```python
from build123d import *

# Parameters (mm, degrees)
BOSS_EXTRUDE1_DEPTH      = 1
F_4_0_4_DIAMETER_HOLE3_D = 4
F_4_0_4_DIAMETER_HOLE2_D = 4
CUT_EXTRUDE1_DEPTH       = 185.301435156
F_4_0_4_DIAMETER_HOLE1_D = 4
LPATTERN1_COUNT          = 10
LPATTERN1_PITCH          = 10
FILLET1_R                = 4


with BuildPart() as part:
    # Sketch1 → Boss-Extrude1 (new body)
    with BuildSketch(Plane(origin=(0, 0, 0), x_dir=(0, 0, -1), z_dir=(1, 0, 0))):
        with BuildLine():
            Line((12, -183), (12, -85))
            ThreePointArc((12, -85), (21.475099597, -58.206374501), (18, -30))
            Line((18, -30), (18, 0))
            Line((18, 0), (-18, 0))
            Line((-18, 0), (-18, -30))
            ThreePointArc((-18, -30), (-21.475099597, -58.206374501), (-12, -85))
            Line((-12, -85), (-12, -183))
            Line((-12, -183), (12, -183))
        make_face()
    extrude(amount=BOSS_EXTRUDE1_DEPTH)

    # Ø4.0 (4) Diameter Hole3 (through all)
    with Locations(Plane.ZY):
        with Locations((10, -10), (-10, -10)):
            Hole(F_4_0_4_DIAMETER_HOLE3_D / 2)

    # Ø4.0 (4) Diameter Hole2 (through all)
    with Locations(Plane.ZY):
        with Locations((-13, -19), (13, -19)):
            Hole(F_4_0_4_DIAMETER_HOLE2_D / 2)

    # Sketch10 → Cut-Extrude1 (cut, through all)
    with BuildSketch(Plane(origin=(1, 0, 0), x_dir=(0, 0, -1), z_dir=(1, 0, 0))):
        with BuildLine():
            Line((-2, -15), (2, -15))
            ThreePointArc((2, -15), (3, -16), (2, -17))
            Line((2, -17), (-2, -17))
            ThreePointArc((-2, -17), (-3, -16), (-2, -15))
        make_face()
    extrude(amount=-CUT_EXTRUDE1_DEPTH, mode=Mode.SUBTRACT)

    # Ø4.0 (4) Diameter Hole1 (through all)
    with Locations(Plane(origin=(1, 0, 0), x_dir=(0, 0, -1), z_dir=(1, 0, 0))):
        with Locations((-6, -177), (6, -177)):
            f_4_0_4_diameter_hole1 = Hole(F_4_0_4_DIAMETER_HOLE1_D / 2)

    # LPattern1: Ø4.0 (4) Diameter Hole1 ×10
    with Locations(*[(0, i * LPATTERN1_PITCH, 0) for i in range(1, LPATTERN1_COUNT)]):
        add(f_4_0_4_diameter_hole1, mode=Mode.SUBTRACT)

    # Fillet1
    fillet1_edges = [part.edges().sort_by_distance(p)[0] for p in [
        (0.5, 0, 18),
        (0.5, 0, -18),
        (0.5, -183, -12),
        (0.5, -183, 12),
    ]]
    fillet(fillet1_edges, radius=FILLET1_R)


solid = part.part
```
Source: CAD feature listing. Evaluate the final solid. Frame: model axes, mm. Give positions to 0.01 mm unless a question says otherwise; leave off trailing zeros. Loops run counter-clockwise (first coordinate to the right, second up) from the corner with the lowest first, then second, coordinate; pieces in that order, holes last. Notation, with made-up numbers: (-4.75, 57.5) - (21.25, 57.5) arc R27 cw to (21.25, 77.5) - close; hole circle Ø4 at (78.25, 83.5). An arc over 180 degrees is marked (long way). Use CSV: the item, a comma, the result in double quotes.
1) Cut plane D-D (y = -132.5). Output: boundary loops of the cut face in (x, z).
Worked out:
outline,"(0, -12) - (1, -12) - (1, 12) - (0, 12) - close"
2) Cut plane A-A (y = -19). Output: boundary loops of the cut face in (x, z).
Worked out:
outline,"(0, -18) - (1, -18) - (1, -15) - (0, -15) - close; (0, -11) - (1, -11) - (1, 11) - (0, 11) - close; (0, 15) - (1, 15) - (1, 18) - (0, 18) - close"
3) Mould query, pull axis Y, two halves, no side actions, for faces 1 (the cylindrical face through (0.507, -181.797, -10.859)), 2 (the cylindrical face through (0.493, -115.314, -4.925)), 3 (the cylindrical face through (0.493, -57.807, 21.517)), 4 (the cylindrical face through (0.493, -168.774, 6.923)). Classes: +Y half, -Y half, draft (parallel to the pull), parting line (faces both ways), or undercut.
Worked out:
face 1,"-Y half"
face 2,"undercut"
face 3,"parting line"
face 4,"undercut"
4) Cut plane B-B (x = 0.2). Count the separate pieces of the cut face and the enclosed holes in it, and give its area (3 significant figures).
Worked out:
separate pieces,"1"
enclosed holes,"25"
area,"5,240 mm^2"
5) Cut plane C-C (y = -177). Output: boundary loops of the cut face in (x, z), and give its area (3 significant figures).
Worked out:
outline,"(0, -12) - (1, -12) - (1, -8) - (0, -8) - close; (0, -4) - (1, -4) - (1, 4) - (0, 4) - close; (0, 8) - (1, 8) - (1, 12) - (0, 12) - close"
area,"16.0 mm^2"
6) Line query: line 1 (Z direction, x = 0.4, y = -157); line 2 (Z direction, x = 0.85, y = -172.5); line 3 (Y direction, x = 0.55, z = 12.5). Output: solid intervals per line, ascending.
Worked out:
line 1,"z = -12 to -8, -4 to 4, 8 to 12"
line 2,"z = -12 to 12"
line 3,"y = -84.21 to -20.94, -17.06 to 0"
